Geometry check sheet. Reference: drawing and pictorial views, mm from the part's lowest x, y, z. A direction names the side the tool comes from. Give positions to 0.01 mm unless a question says otherwise; leave off trailing zeros. Loops run counter-clockwise (first coordinate to the right, second up) from the corner with the lowest first, then second, coordinate; pieces in that order, holes last. Notation, with made-up numbers: M 87,-31.75 L 116,-31.75 A18 cw 116,-22.75 Z; hole C 7,31 d7. An arc over 180 degrees is marked long. One line per question, with ' | ' between items. Start each with the question number.
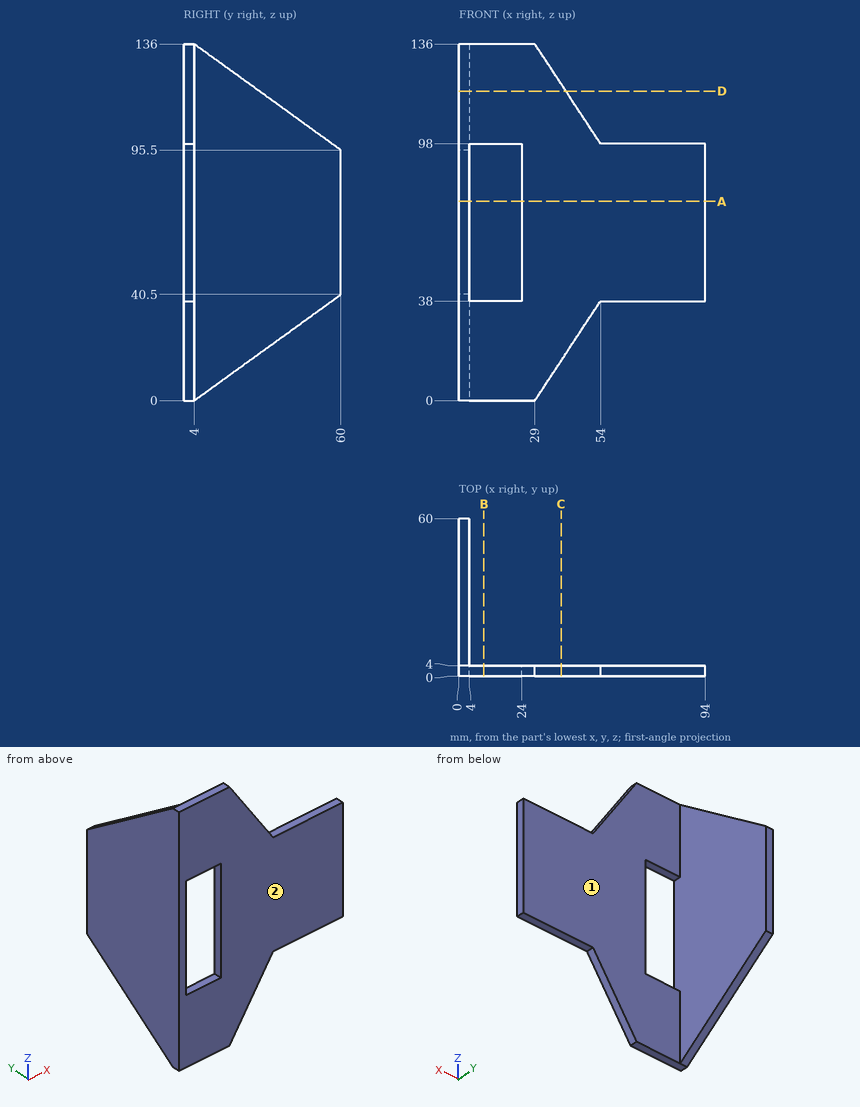
Q1. Cross-section at B-B (x = 9.5). Record the cut outline in (y, z).
Q2. Cross-section at D-D (z = 118). Record the cut outline in (x, y), and give its area (3 significant figures).
Q3. Material ranges on probe 1 along Y at (x, z) = (90.5, 95.5), recorded low to high. Write a range as from..to.
Q4. Access from +Z, -Z, +X, -X, +Y, -Y to the whole of each face (thin tool, end or side, straight path). Record for the marked faces 1 and 2.
Q5. Depth check by flat-ended pin: P1, Ø1.5, axis at y = 44, z = 101.5, coming from the -X side; P2, Ø6, axis at y = 13, z = 16, coming from the +X side; P3, Ø1.5, axis at x = 54.5, z = 65, coming from the +Y side; P4, Ø3, axis at x = 73.5, y = 3, coming from the -Z side. Enter the tip coordinate at first touch or a pass-through.
Q6. Cross-section at A-A (z = 76). Record the cut outline in (x, y), and give its area (3 significant figures).
Q7. Cross-section at C-C (x = 39). Record the cut outline in (y, z).
Solved:
1) outline: M 0,0 L 4,0 L 4,38 L 0,38 Z; M 0,98 L 4,98 L 4,136 L 0,136 Z
2) outline: M 0,0 L 40.84,0 L 40.84,4 L 4,4 L 4,28.89 L 0,28.89 Z | area: 263 mm²
3) probe 1: y = 0..4
4) face 1: +Z, -Z, +X, +Y | face 2: +Z, -Z, +X, -X, -Y
5) P1: stops at x = 0 | P2: stops at x = 4 | P3: stops at y = 4 | P4: stops at z = 38
6) outline: M 0,0 L 4,0 L 4,60 L 0,60 Z; M 24,0 L 94,0 L 94,4 L 24,4 Z | area: 520 mm²
7) outline: M 0,15.2 L 4,15.2 L 4,120.8 L 0,120.8 Z
